CAD build for the part. Positions are in the model's coordinates, mm. A direction names the side the tool comes from. Give positions to 0.01 mm unless a question says otherwise; leave off trailing zeros. Write each loop counter-clockwise with the first axis right and the second up, starting at its lowest first coordinate (ties: lowest second). Pieces come first, ordered by that corner, then holes. Notation, with made-up numbers: (68.25, -10.75) -> (126.25, -10.75) arc R22 cw to (126.25, 25.25) -> close; hole circle Ø7 at (52, 42.5). An arc over 180 degrees is marked (long way). Answer as a JSON object with one key per item and string values.
```python
from build123d import *

# Parameters (mm, degrees)
SKETCH_1_R          = 1.85
EXTRUDE_1_DEPTH     = 3.3
SKETCH_2_W          = 3.3
SKETCH_2_H          = 58.544472475
EXTRUDE_2_DEPTH     = 3.3
EXTRUDE_2_2_DEPTH   = 3.3
SKETCH_3_W          = 47.8
SKETCH_3_H          = 17.46
EXTRUDE_3_DEPTH     = 3.3
SKETCH_4_W          = 28
SKETCH_4_H          = 28
CUT_EXTRUDE_2_DEPTH = 3.3
SKETCH_5_R          = 1.8
SKETCH_5_R_2        = 1.3
EXTRUDE_4_DEPTH     = 1.6


with BuildPart() as part:
    # Sketch 1 → Extrude 1 (new body)
    with BuildSketch(Plane.XY):
        Polygon((21.926158038, 28.738964578), (21.926158038, -28.626702997), (-19.273841962, -28.626702997), (-19.273841962, 28.738964578), (-19.273841962, 29.888964578), (21.926158038, 29.888964578), align=None)
        with Locations((11.226158038, -8.761035422)):
            Circle(SKETCH_1_R, mode=Mode.SUBTRACT)
        with Locations((-9.7, -8.761035422)):
            Circle(SKETCH_1_R, mode=Mode.SUBTRACT)
    extrude(amount=-EXTRUDE_1_DEPTH)


with BuildPart() as body_2:
    # Sketch 2 → Extrude 2 (new body)
    with BuildSketch(Plane.XY):
        with Locations((23.576158038, 0.61672834)):
            Rectangle(SKETCH_2_W, SKETCH_2_H)
    extrude(amount=-EXTRUDE_2_DEPTH)



with BuildPart() as body_3:
    # Sketch 2 → Extrude 2 2 (new body)
    with BuildSketch(Plane.XY):
        with Locations((-20.923841962, 0.61672834)):
            Rectangle(SKETCH_2_W, SKETCH_2_H)
    extrude(amount=-EXTRUDE_2_2_DEPTH)


with BuildPart() as body_2_1:
    add(body_2.part)

    add(body_3.part)  # Extrude 3 merges body 3
    # Sketch 3 → Extrude 3 (add)
    with BuildSketch(Plane.XY):
        with Locations((1.326158038, -37.385507897)):
            Rectangle(SKETCH_3_W, SKETCH_3_H)
    extrude(amount=-EXTRUDE_3_DEPTH)


with BuildPart() as cut_extrude_2_tool:
    # Sketch 4 → Cut-Extrude 2 (new body)
    with BuildSketch(Plane.XY):
        with Locations((1.326158038, -27.495005481)):
            Rectangle(SKETCH_4_W, SKETCH_4_H)
        with Locations((1.326158038, 11.379364932)):
            Rectangle(SKETCH_4_W, SKETCH_4_H)
    extrude(amount=-CUT_EXTRUDE_2_DEPTH)


with BuildPart() as part_1:
    add(part.part)

    # Cut-Extrude 2: cut by cut_extrude_2_tool
    add(cut_extrude_2_tool.part, mode=Mode.SUBTRACT)



with BuildPart() as body_2_2:
    add(body_2_1.part)

    # Cut-Extrude 2: cut by cut_extrude_2_tool
    add(cut_extrude_2_tool.part, mode=Mode.SUBTRACT)


with BuildPart() as part_2:
    add(part_1.part)

    add(body_2_2.part)  # Extrude 4 merges body 2
    # Sketch 5 → Extrude 4 (add)
    with BuildSketch(Plane.XY):
        with Locations((-23.173841962, 39.740306118)):
            Circle(SKETCH_5_R)
        with Locations((-23.173841962, 39.740306118)):
            Circle(SKETCH_5_R_2, mode=Mode.SUBTRACT)
        with BuildLine():
            Line((-24.920422623, 39.305040689), (-22.573841962, 29.888964578))
            Line((-22.573841962, 29.888964578), (-19.273841962, 29.888964578))
            Line((-19.273841962, 29.888964578), (-21.411987289, 40.108909035))
            ThreePointArc((-21.411987289, 40.108909035), (-21.38340369, 39.925591827), (-21.373841962, 39.740306118))
            ThreePointArc((-21.373841962, 39.740306118), (-22.954576359, 37.953710866), (-24.920422623, 39.305040689))
        make_face()
        with BuildLine():
            ThreePointArc((27.626158038, 39.740306118), (25.826158038, 41.540306118), (24.026158038, 39.740306118))
            ThreePointArc((24.026158038, 39.740306118), (25.400100428, 37.991456521), (27.424463497, 38.912405363))
            Line((27.424463497, 38.912405363), (27.626158038, 39.740306118))
        make_face()
        with Locations((25.826158038, 39.740306118)):
            Circle(SKETCH_5_R_2, mode=Mode.SUBTRACT)
        with BuildLine():
            ThreePointArc((27.424463497, 38.912405363), (25.400100428, 37.991456521), (24.026158038, 39.740306118))
            Line((24.026158038, 39.740306118), (21.926158038, 29.888964578))
            Line((21.926158038, 29.888964578), (25.226158038, 29.888964578))
            Line((25.226158038, 29.888964578), (27.424463497, 38.912405363))
        make_face()
        with Locations((-23.173841962, -18.259693882)):
            Circle(SKETCH_5_R)
        with Locations((-23.173841962, -18.259693882)):
            Circle(SKETCH_5_R_2, mode=Mode.SUBTRACT)
        with Locations((25.826158038, -18.259693882)):
            Circle(SKETCH_5_R)
        with Locations((25.826158038, -18.259693882)):
            Circle(SKETCH_5_R_2, mode=Mode.SUBTRACT)
    extrude(amount=-EXTRUDE_4_DEPTH)


solid = part_2.part
```
1) Slice it at B-B (x = 8.5). List the corners of the cut face in (y, z) (1 decimal), then the cut area to 3 significant figures.
Model answer:
{"outline": "(-46.1, -3.3) -> (-41.5, -3.3) -> (-41.5, 0) -> (-46.1, 0) -> close; (-13.5, -3.3) -> (-2.6, -3.3) -> (-2.6, 0) -> (-13.5, 0) -> close; (25.4, -3.3) -> (29.9, -3.3) -> (29.9, 0) -> (25.4, 0) -> close", "area": "66.0 mm2"}
2) Slice it at D-D (x = 17.5). List the corners of the cut face in (y, z).
Model answer:
{"outline": "(-46.12, -3.3) -> (-28.66, -3.3) -> (-28.66, 0) -> (-46.12, 0) -> close; (-28.63, -3.3) -> (29.89, -3.3) -> (29.89, 0) -> (-28.63, 0) -> close"}
3) Wall check: probe 1 along Y at (x, z) = (-3.5, -2.85) (1 decimal); probe 2 along Y at (x, z) = (-9.7, -1.9) (1 decimal); probe 3 along X at (y, z) = (-38.5, -2.4). Give the ranges that are in metal, low to high.
Model answer:
{"probe 1": "y = -46.1 to -41.5, -13.5 to -2.6, 25.4 to 29.9", "probe 2": "y = -46.1 to -41.5, -13.5 to -10.6, -6.9 to -2.6, 25.4 to 29.9", "probe 3": "x = -22.57 to -12.67, 15.33 to 25.23"}
4) Slice it at C-C (x = -9.7). List the corners of the cut face in (y, z) (1 decimal), then the cut area to 3 significant figures.
Model answer:
{"outline": "(-46.1, -3.3) -> (-41.5, -3.3) -> (-41.5, 0) -> (-46.1, 0) -> close; (-13.5, -3.3) -> (-10.6, -3.3) -> (-10.6, 0) -> (-13.5, 0) -> close; (-6.9, -3.3) -> (-2.6, -3.3) -> (-2.6, 0) -> (-6.9, 0) -> close; (25.4, -3.3) -> (29.9, -3.3) -> (29.9, 0) -> (25.4, 0) -> close", "area": "53.8 mm2"}
5) Slice it at A-A (y = -36.5). List the corners of the cut face in (x, z).
Model answer:
{"outline": "(-22.57, -3.3) -> (-12.67, -3.3) -> (-12.67, 0) -> (-22.57, 0) -> close; (15.33, -3.3) -> (25.23, -3.3) -> (25.23, 0) -> (15.33, 0) -> close"}
6) 3-axis set-ups, long thin cutter, end or side, ignore diameter. For faces 1 (the flat face through (1, 25.379, -2)), 2 (the flat face through (22.99, 34.88, -0.79)), 3 (the flat face through (1, -11, 0)), 4 (the flat face through (-23.764, 34.663, -0.789)): which of +Z, -Z, +X, -X, +Y, -Y reach the whole face in a straight line?
Model answer:
{"face 1": "+Z, -Z", "face 2": "+Z, -Z, +Y", "face 3": "+Z, +X, -X, +Y, -Y", "face 4": "+Z, -Z, -X"}
7) Pin check, flat tips, straight feed: pin 1 (4.5 mm diameter, centred on x = -9.7, y = -8.76, fed in from -Z); pin 2 (1.5 mm diameter, centred on y = -1.5, z = -3, fed in from +X); pin 3 (1.5 mm diameter, centred on x = -10.5, z = -1, fed in from +Y); pin 4 (1.6 mm diameter, centred on x = 25.83, y = 39.74, fed in from -Z). Stop position of each tip, or through.
Model answer:
{"pin 1": "stops at z = -3.3", "pin 2": "stops at x = 25.23", "pin 3": "stops at y = 29.89", "pin 4": "passes through"}
